Read the model definition and answer for the solid it produces. Units are mm, in the model's axes. Coordinates: 2 decimals unless noted, no trailing zeros. Order: outer loops, then holes, each group sorted by start corner. A loop starts at its lowest first (then second) coordinate and runs counter-clockwise, first axis right, second up. Notation, with made-up numbers: (-35, 34) - (-19, 34) arc R11 ccw to (-19, 53) - close; hole circle Ø10 at (27.25, 25). An arc over 180 degrees is marked (long way). Write item = value, one per line.
from build123d import *

# Parameters (mm, degrees)
BOSS_EXTRUDE1_DEPTH = 4
CUT_EXTRUDE1_DEPTH  = 1
SKETCH4_R           = 1.6
CUT_EXTRUDE2_DEPTH  = 10
BOSS_EXTRUDE2_START = 1
SKETCH6_R           = 1.6
BOSS_EXTRUDE2_DEPTH = 1
SKETCH7_W           = 20
SKETCH7_H           = 4
BOSS_EXTRUDE3_DEPTH = 85.1


with BuildPart() as part:
    # Sketch1 → Boss-Extrude1 (new body)
    with BuildSketch(Plane(origin=(0, 0, 0), x_dir=(1, 0, 0), z_dir=(0, 1, 0))):
        with BuildLine():
            Line((-10, -15), (-10, -34.803693177))
            Line((-10, -34.803693177), (10, -34.803693177))
            Line((10, -34.803693177), (10, -15))
            ThreePointArc((10, -15), (10.472630633, -11.957512347), (11.845976177, -9.201785066))
            ThreePointArc((11.845976177, -9.201785066), (0, 15), (-11.845976177, -9.201785066))
            ThreePointArc((-11.845976177, -9.201785066), (-10.472630633, -11.957512347), (-10, -15))
        make_face()
    extrude(amount=BOSS_EXTRUDE1_DEPTH)

    # Sketch2 → Cut-Revolve1 (revolve, cut)
    with BuildSketch(Plane(origin=(0, 4, 0), x_dir=(1, 0, 0), z_dir=(0, 1, 0))):
        with BuildLine():
            Line((0, 10.1), (0, -10.1))
            ThreePointArc((0, -10.1), (10.1, 0), (0, 10.1))
        make_face()
    revolve(axis=Axis((0, 4, -10.1), (0, 0, 1)), mode=Mode.SUBTRACT)

    # Sketch3 → Cut-Extrude1 (cut)
    with BuildSketch(Plane(origin=(0, 4, 0), x_dir=(1, 0, 0), z_dir=(0, 1, 0))):
        with BuildLine():
            Line((10, -24.901846588), (10, -39.974302239))
            ThreePointArc((10, -39.974302239), (0, -49.974302239), (-10, -39.974302239))
            Line((-10, -39.974302239), (-10, -24.901846588))
            ThreePointArc((-10, -24.901846588), (0, -14.901846588), (10, -24.901846588))
        make_face()
    extrude(amount=-CUT_EXTRUDE1_DEPTH, mode=Mode.SUBTRACT)

    # Sketch4 → Cut-Extrude2 (cut)
    with BuildSketch(Plane(origin=(0, 3, 0), x_dir=(1, 0, 0), z_dir=(0, 1, 0))):
        with Locations(Location((5, -24.901846588, 0), (0, 0, 270))):
            Circle(SKETCH4_R)
        with Locations(Location((-5, -24.901846588, 0), (0, 0, 90))):
            Circle(SKETCH4_R)
    extrude(amount=-CUT_EXTRUDE2_DEPTH, mode=Mode.SUBTRACT)

    # Sketch6 → Boss-Extrude2 (add)
    with BuildSketch(Plane(origin=(0, 3, 0), x_dir=(1, 0, 0), z_dir=(0, 1, 0)).offset(BOSS_EXTRUDE2_START)):
        with BuildLine():
            Line((-10, -24.901846588), (-10, -34.803693177))
            Line((-10, -34.803693177), (10, -34.803693177))
            Line((10, -34.803693177), (10, -24.901846588))
            ThreePointArc((10, -24.901846588), (0, -14.901846588), (-10, -24.901846588))
        make_face()
        with Locations(Location((-5, -24.901846588, 0), (0, 0, 90))):
            Circle(SKETCH6_R, mode=Mode.SUBTRACT)
        with Locations(Location((5, -24.901846588, 0), (0, 0, 90))):
            Circle(SKETCH6_R, mode=Mode.SUBTRACT)
    extrude(amount=-BOSS_EXTRUDE2_DEPTH)

    # Sketch7 → Boss-Extrude3 (add)
    with BuildSketch(Plane.XY.offset(34.803693177)):
        with Locations((0, 2)):
            Rectangle(SKETCH7_W, SKETCH7_H)
    extrude(amount=BOSS_EXTRUDE3_DEPTH)

    # Mirror3: part across plane


with BuildPart() as part_1:
    add(part.part)
    add(part.part.mirror(Plane(origin=(0, 0, 119.903693177), x_dir=(1, 0, 0), z_dir=(0, 0, -1))))


solid = part_1.part
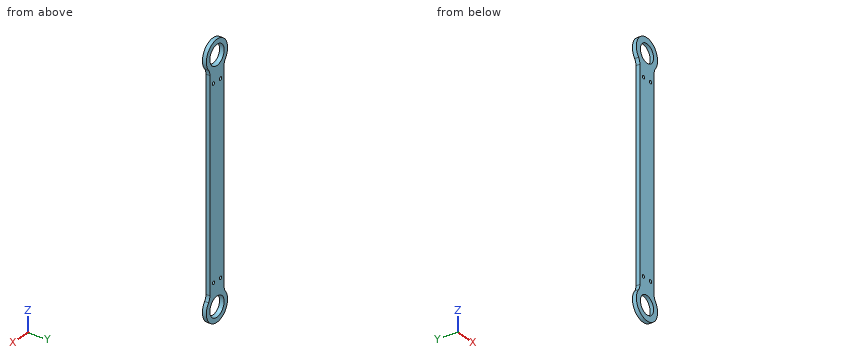
1) Flat-ended cylindrical pins translate along their axes: pin 1 Ø1 at (x, y) = (12, 3.5) entering from -Z; pin 2 Ø2 at (y, z) = (1.5, 23.5) entering from +X; pin 3 Ø1.5 at (x, y) = (-10.5, 3) entering from +Z. Find the tip coordinate at first contact, or state that the pin passes through.
Returned:
pin_1 = -9.63
pin_2 = 10
pin_3 = 251.21
2) The part is cut by section B-B (y = 1.6). Determine the outline of the cut face in (x, z), and give its area (3 significant figures).
Returned:
outline = (-11.85, 9.2) arc R15 ccw (long way) to (11.85, 9.2) arc R10.03 cw to (10, 15) - (10, 224.81) arc R10.03 cw to (11.85, 230.61) arc R15 ccw (long way) to (-11.85, 230.61) arc R10.03 cw to (-10, 224.81) - (-10, 15) arc R10.03 cw to start; hole circle Ø19.62 at (0, 0); hole circle Ø19.62 at (0, 239.81); hole circle Ø3.2 at (-5, 24.9); hole circle Ø3.2 at (-5, 214.91); hole circle Ø3.2 at (5, 24.9); hole circle Ø3.2 at (5, 214.91)
area = 5,030 mm^2
3) Straight lines are drawn through the part: line 1 along Z through (x, y) = (5, 2.4); line 2 along Z through (x, y) = (-5, 2.95); line 3 along Z through (x, y) = (-1.5, 1.3). For each, find the intervals that lie inside material, in ascending order. Write a range as from..to.
Returned:
line_1 = -14.14..-8.63, 8.63..23.3, 26.5..213.31, 216.51..231.18, 248.44..253.95
line_2 = -14.14..-8.71, 8.71..23.3, 26.5..213.31, 216.51..231.09, 248.52..253.95
line_3 = -14.92..-9.62, 9.62..230.19, 249.42..254.73
4) The part is cut by section A-A (z = 0). Determine the outline of the cut face in (x, y), and give its area (3 significant figures).
Returned:
outline = (-15, 0) - (-9.27, 0) arc R10.1 cw to (-10.1, 4) - (-15, 4) - close; (9.27, 0) - (15, 0) - (15, 4) - (10.1, 4) arc R10.1 cw to start
area = 41.4 mm^2
5) The part is cut by section C-C (x = 0). Determine the outline of the cut face in (y, z), and give its area (3 significant figures).
Returned:
outline = (0, -15) - (4, -15) - (4, -10.1) arc R10.1 cw to (0, -9.27) - close; (0, 9.27) arc R10.1 cw to (4, 10.1) - (4, 229.71) arc R10.1 cw to (0, 230.53) - close; (0, 249.08) arc R10.1 cw to (4, 249.91) - (4, 254.81) - (0, 254.81) - close
area = 922 mm^2
6) The part is cut by section D-D (z = 191). Determine the outline of the cut face in (x, y), and give its area (3 significant figures).
Returned:
outline = (-10, 0) - (10, 0) - (10, 4) - (-10, 4) - close
area = 80.0 mm^2
